Autodesk Fusion 360 part; units mm, degrees
sketch "Sketch1" plane through (0, 0, 0) normal (0, 1, 0) x (1, 0, 0)
  circle A0 centre (0, 0) radius 102
  dimension "d1" = 204
extrude "Extrude1" add sketch "Sketch1" along normal blind 6
sketch "Sketch2" plane through (0, 0, 0) normal (0, -1, 0) x (1, 0, 0)
  circle A0 centre (0, 0) radius 102
  circle A1 centre (0, 0) radius 102
  circle A2 centre (0, 0) radius 90
  dimension "d4" = 204
  dimension "d5" = 180
extrude "Extrude2" add sketch "Sketch2" along normal blind 3.5
sketch "Sketch3" plane through (0, -3.5, 0) normal (0, -1, 0) x (1, 0, 0)
  circle A0 centre (0, 0) radius 90
  circle A1 centre (0, 0) radius 102
  circle A2 centre (0, 0) radius 96 construction
  line L0 (0, 0) -> (-67.8823, 67.8823) construction
  line L1 (0, 0) -> (96, 0) construction
  line L2 (0, 0) -> (67.8823, 67.8823) construction
  line L3 (0, 0) -> (96, 0) construction
  line L4 (0, 0) -> (-67.8823, -67.8823) construction
  line L5 (0, 0) -> (96, 0) construction
  line L6 (0, 0) -> (67.8823, -67.8823) construction
  line L7 (0, 0) -> (96, 0) construction
  circle A3 centre (-67.8823, 67.8823) radius 2.925
  circle A4 centre (67.8823, 67.8823) radius 2.925
  circle A5 centre (-67.8823, -67.8823) radius 2.925
  circle A6 centre (67.8823, -67.8823) radius 2.925
  dimension "d8" = 192
  dimension "d9" = 135
  dimension "d10" = 45
  dimension "d11" = 135
  dimension "d12" = 45
  dimension "d13" = 5.85
  dimension "d14" = 5.85
  dimension "d15" = 5.85
  dimension "d16" = 5.85
extrude "Extrude3" add sketch "Sketch3" along normal blind 2.5 contours A3 | A4 | A5 | A6
sketch "Sketch4" plane through (0, 6, 0) normal (0, 1, 0) x (-1, 0, 0)
  circle A0 centre (0, 0) radius 102
  line L0 (0, 0) -> (0, -64) construction
  line L1 (40, -81.5) -> (-40, -81.5)
  line L2 (-40, -81.5) -> (-40, -46.5)
  line L3 (-40, -46.5) -> (40, -46.5)
  line L4 (40, -46.5) -> (40, -81.5)
  line L5 (40, -81.5) -> (-40, -46.5) construction
  line L6 (-40, -81.5) -> (40, -46.5) construction
  point P0 (0, -64)
  dimension "d19" = 64
  dimension "d20" = 80
  dimension "d21" = 35
extrude "Extrude4" cut sketch "Sketch4" against normal blind 20 contours L1 L2 L3 L4
sketch "Sketch5" plane through (0, 6, 0) normal (0, 1, 0) x (-1, 0, 0)
  line L0 (-40, -81.5) -> (-40, -46.5)
  line L1 (-40, -46.5) -> (40, -46.5)
  line L2 (40, -46.5) -> (40, -81.5)
  line L3 (40, -81.5) -> (-40, -81.5)
  circle A0 centre (0, 0) radius 102
  line L4 (40, 0) -> (-40, 0)
  arc A1 (40, 0) -> (-40, 0) centre (0, 0) ccw
  circle A2 centre (0, 0) radius 70 construction
  line L5 (0, 0) -> (49.4975, -49.4975) construction
  line L6 (0, 0) -> (70, 0) construction
  line L7 (0, 0) -> (49.4975, 49.4975) construction
  line L8 (0, 0) -> (70, 0) construction
  line L9 (0, 0) -> (-49.4975, -49.4975) construction
  line L10 (0, 0) -> (70, 0) construction
  line L11 (0, 0) -> (-49.4975, 49.4975) construction
  line L12 (0, 0) -> (70, 0) construction
  line L13 (0, 0) -> (98, 0) construction
  line L14 (0, 0) -> (98, 0) construction
  line L15 (0, 0) -> (98, 0) construction
  line L16 (-82.693, 30.0978) -> (-92.0899, 33.518)
  line L17 (0, 0) -> (98, 0) construction
  line L18 (30.0978, 82.693) -> (33.518, 92.0899)
  line L19 (0, 0) -> (98, 0) construction
  line L20 (-30.0978, 82.693) -> (-33.518, 92.0899)
  line L21 (0, 0) -> (98, 0) construction
  line L22 (82.693, -30.0978) -> (92.0899, -33.518)
  line L23 (82.693, 30.0978) -> (92.0899, 33.518)
  line L24 (-82.693, -30.0978) -> (-92.0899, -33.518)
  line L25 (60.1951, -64.1915) -> (74.0503, -64.1915)
  line L26 (-60.1951, -64.1915) -> (-74.0503, -64.1915)
  arc A3 (-74.0503, -64.1915) -> (74.0503, -64.1915) centre (0, 0) ccw
  arc A4 (-82.693, 30.0978) -> (-82.693, -30.0978) centre (0, 0) ccw
  arc A5 (-92.0899, 33.518) -> (-92.0899, -33.518) centre (0, 0) ccw
  arc A6 (92.0899, -33.518) -> (92.0899, 33.518) centre (0, 0) ccw
  arc A7 (33.518, 92.0899) -> (-33.518, 92.0899) centre (0, 0) ccw
  arc A8 (82.693, -30.0978) -> (82.693, 30.0978) centre (0, 0) ccw
  arc A9 (30.0978, 82.693) -> (-30.0978, 82.693) centre (0, 0) ccw
  line L27 (-60.1951, -64.1915) -> (-40, -64.1915)
  line L28 (40, -64.1915) -> (60.1951, -64.1915)
  circle A10 centre (49.4975, -49.4975) radius 1.5
  circle A11 centre (49.4975, -49.4975) radius 3
  circle A12 centre (-49.4975, -49.4975) radius 1.5
  circle A13 centre (-49.4975, -49.4975) radius 3
  circle A14 centre (49.4975, 49.4975) radius 1.5
  circle A15 centre (49.4975, 49.4975) radius 3
  circle A16 centre (-49.4975, 49.4975) radius 1.5
  circle A17 centre (-49.4975, 49.4975) radius 3
  dimension "d24" = 176
  dimension "d25" = 196
  dimension "d26" = 80
  dimension "d27" = 140
  dimension "d28" = 45
  dimension "d29" = 45
  dimension "d30" = 135
  dimension "d31" = 135
  dimension "d35" = 160
  dimension "d36" = 70
  dimension "d37" = 110
  dimension "d38" = 3
  dimension "d39" = 6
  dimension "d40" = 3
  dimension "d41" = 6
  dimension "d42" = 3
  dimension "d43" = 6
  dimension "d44" = 3
  dimension "d45" = 6
extrude "Extrude5" cut sketch "Sketch5" against normal blind 20 contours A10 | A12 | A14 | A16
extrude "Extrude6" cut sketch "Sketch5" against normal blind 4 contours A11 | A13 | A15 | A17
extrude "Extrude7" add sketch "Sketch5" along normal blind 10 contours L0 L2 L3 L25 L26 A3 L27 L28 | L4 A1 | L16 L24 A4 A5 | L18 L20 A7 A9 | L22 L23 A6 A8
sketch "Sketch6" plane through (0, 16, 0) normal (0, 1, 0) x (-1, 0, 0)
  arc A0 (40, 0) -> (-40, 0) centre (0, 0) ccw
  line L0 (-40, 0) -> (40, 0)
  circle A1 centre (0, 0) radius 93 construction
  circle A2 centre (0, 0) radius 20 construction
  line L1 (0, 0) -> (0, 20) construction
  line L2 (0, 0) -> (91.5871, -16.1493) construction
  line L3 (0, 0) -> (93, 0) construction
  line L4 (0, 0) -> (91.5871, 16.1493) construction
  line L5 (0, 0) -> (93, 0) construction
  line L6 (0, 0) -> (-91.5871, -16.1493) construction
  line L7 (0, 0) -> (93, 0) construction
  line L8 (0, 0) -> (-91.5871, 16.1493) construction
  line L9 (0, 0) -> (93, 0) construction
  line L10 (0, 0) -> (16.1493, 91.5871) construction
  line L11 (0, 0) -> (93, 0) construction
  line L12 (0, 0) -> (-16.1493, 91.5871) construction
  line L13 (0, 0) -> (93, 0) construction
  line L14 (0, 0) -> (0, -93) construction
  line L15 (0, 0) -> (-53.3426, -76.1811) construction
  line L16 (0, 0) -> (53.3426, -76.1811) construction
  circle A3 centre (0, -93) radius 3
  circle A4 centre (-53.3426, -76.1811) radius 3
  circle A5 centre (53.3426, -76.1811) radius 3
  circle A6 centre (91.5871, -16.1493) radius 3
  circle A7 centre (91.5871, 16.1493) radius 3
  circle A8 centre (-91.5871, -16.1493) radius 3
  circle A9 centre (-91.5871, 16.1493) radius 3
  circle A10 centre (-16.1493, 91.5871) radius 3
  circle A11 centre (16.1493, 91.5871) radius 3
  circle A12 centre (0, 20) radius 3
  dimension "d52" = 186
  dimension "d53" = 40
  dimension "d54" = 10
  dimension "d55" = 10
  dimension "d56" = 170
  dimension "d57" = 170
  dimension "d58" = 80
  dimension "d59" = 100
  dimension "d60" = 145
  dimension "d61" = 6
  dimension "d62" = 6
  dimension "d63" = 6
  dimension "d64" = 6
  dimension "d65" = 6
  dimension "d66" = 6
  dimension "d67" = 6
  dimension "d68" = 6
  dimension "d69" = 6
  dimension "d70" = 6
extrude "Extrude8" cut sketch "Sketch6" against normal blind 3.2 contours A3 | A4 | A5 | A6 | A7 | A8 | A9 | A10 | A11 | A12
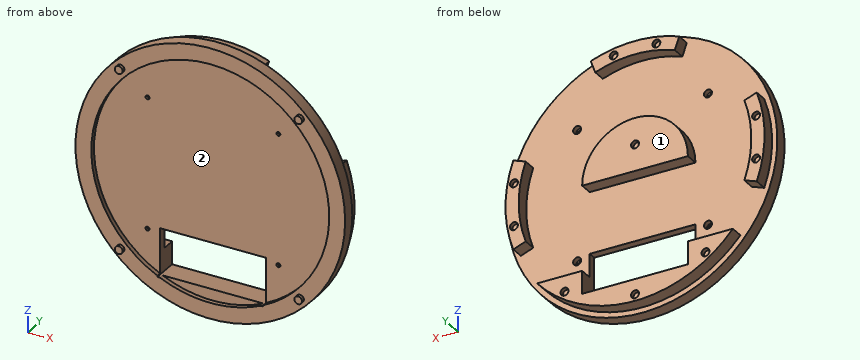
Verification items for the finished model (mm, model axes). Face numbers are marked on the shaded views. Coordinates: 2 decimals unless noted, no trailing zeros. Write each loop counter-clockwise with the first axis right and the second up, starting at its lowest first coordinate (ties: lowest second). Pieces come first, ordered by that corner, then holes. Notation, with made-up numbers: (12, -0.75) - (52, -0.75) arc R26 ccw to (52, 23.25) - close; hole circle Ø10 at (-19, 48.5). An arc over 180 degrees is marked (long way). Answer as a JSON object with one key per item and string values.
(1) Gauge pin test, flat ends, axial feed: pin 1 Ø5.5 at (x, z) = (-91.59, -16.15) entering from +Y; pin 2 Ø8 at (x, z) = (53.34, -76.18) entering from -Y; pin 3 Ø5 at (x, y) = (6.5, 4.5) entering from -Z; pin 4 Ø1.8 at (x, z) = (-49.5, -50) entering from +Y. Record the tip position at first contact, or that the pin passes through.
Report:
{"pin 1": "y = 12.8", "pin 2": "y = -3.5", "pin 3": "z = -101.92", "pin 4": "through"}
(2) Cross-section at B-B on y = 9. Record the cut outline in (x, z), plus the area to 3 significant figures.
Report:
{"outline": "(-92.09, -33.52) - (-82.69, -30.1) arc R88 cw to (-82.69, 30.1) - (-92.09, 33.52) arc R98 ccw to start; (-74.05, -64.19) arc R98 ccw to (74.05, -64.19) - (40, -64.19) - (40, -81.5) - (-40, -81.5) - (-40, -64.19) - close; (-40, 0) - (40, 0) arc R40 ccw to start; (-33.52, 92.09) - (-30.1, 82.69) arc R88 cw to (30.1, 82.69) - (33.52, 92.09) arc R98 ccw to start; (82.69, -30.1) - (92.09, -33.52) arc R98 ccw to (92.09, 33.52) - (82.69, 30.1) arc R88 cw to start", "area": "6,550 mm^2"}
(3) Thickness scan on line 1 along X through (y, z) = (7, 1.5); line 2 along Z through (x, y) = (-2, -0.75); line 3 along X through (y, z) = (-2.25, 1). Record the ranges inside material, lowest first.
Report:
{"line 1": "-97.99 to -87.99, -39.97 to 39.97, 87.99 to 97.99", "line 2": "-101.98 to -89.98, 89.98 to 101.98", "line 3": "-102 to -89.99, 89.99 to 102"}
(4) Cross-section at C-C on z = -39. Record the cut outline in (x, y), plus the area to 3 significant figures.
Report:
{"outline": "(-94.25, -3.5) - (-81.11, -3.5) - (-81.11, 0) - (81.11, 0) - (81.11, -3.5) - (94.25, -3.5) - (94.25, 6) - (-94.25, 6) - close", "area": "1,220 mm^2"}
(5) Mould release check, pull along X, two halves, no side actions. Record for the marked faces 1 and 2: pulls with the +X half, pulls with the -X half, needs draft (parallel to the pull), parting line crosses it, or undercut.
Report:
{"face 1": "needs draft", "face 2": "undercut"}
(6) Cross-section at D-D on z = -93. Record the cut outline in (x, y).
Report:
{"outline": "(-41.89, -3.5) - (41.89, -3.5) - (41.89, 6) - (30.9, 6) - (30.9, 16) - (3, 16) - (3, 12.8) - (-3, 12.8) - (-3, 16) - (-30.9, 16) - (-30.9, 6) - (-41.89, 6) - close"}
